Geometry: see drawing. Coordinates: mm, zero at the bounding-box minimum. A direction names the side the tool comes from. Coordinates: 2 decimals unless noted, no trailing zeros. Order: outer loops, then holes, each group sorted by start corner. A loop starts at its lowest first (then second) coordinate and runs counter-clockwise, first axis right, second up.
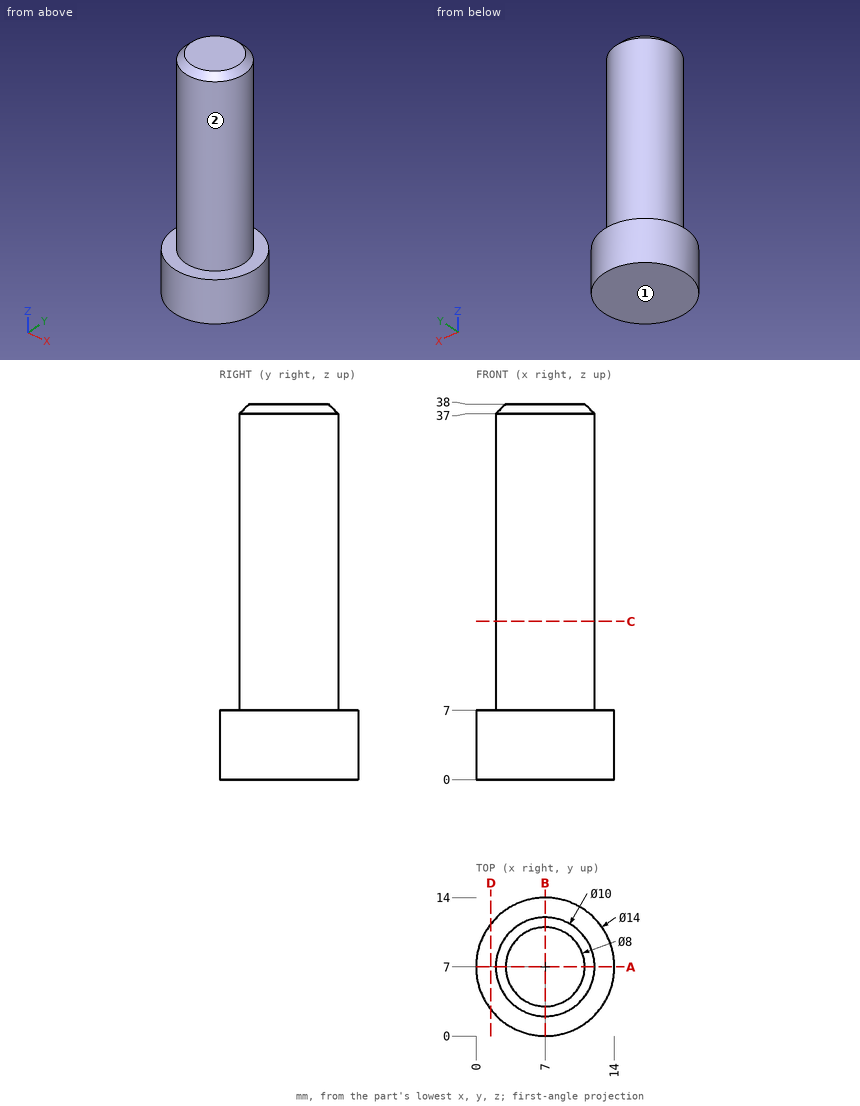
Q1. Set-up query: the marked faces 1 and 2. Return all of +Z, -Z, +X, -X, +Y, -Y with unobstructed straight access to the full face (end or side cutting, diameter ignored); none if empty.
Solutions:
face 1: -Z, +X, -X, +Y, -Y
face 2: +Z
Q2. Section query D-D on x = 1.5. Output: boundary loops of the cut face in (y, z).
Solutions:
outline: (2.67, 0) - (11.33, 0) - (11.33, 7) - (2.67, 7) - close
Q3. Pin query (flat end, axial travel): P1, Ø8, axis at x = 3.5, y = 7, coming from the -Z side; P2, Ø2, axis at y = 9, z = 26.5, coming from the +X side; P3, Ø1.5, axis at y = 9.5, z = 15.5, coming from the -X side; P4, Ø8, axis at y = 9.5, z = 30.5, coming from the -X side. Return the tip coordinate at first contact, or that it passes through.
Solutions:
P1: stops at z = 0
P2: stops at x = 11.9
P3: stops at x = 2.32
P4: stops at x = 2
Q4. Section query C-C on z = 16. Output: boundary loops of the cut face in (x, y).
Solutions:
outline: circle Ø10 at (7, 7)
Q5. Material intervals for line 1 along Y through (x, z) = (7, 19.5); line 2 along X through (y, z) = (4, 20.5); line 3 along Z through (x, y) = (4.75, 2), sorted ascending.
Solutions:
line 1: y = 2 to 12
line 2: x = 3 to 11
line 3: z = 0 to 7
Q6. Section query A-A on y = 7. Output: boundary loops of the cut face in (x, z), plus the area to 3 significant figures.
Solutions:
outline: (0, 0) - (14, 0) - (14, 7) - (12, 7) - (12, 37) - (11, 38) - (3, 38) - (2, 37) - (2, 7) - (0, 7) - close
area: 407 mm2
